Check sheet for the modelled part. Datum: model origin and axes. Units: mm. Round coordinates to 2 decimals unless told otherwise and drop trailing zeros. Write each loop counter-clockwise with the first axis right and the second up, starting at its lowest first coordinate (ties: lowest second). Pieces come first, ordered by that corner, then holes. Notation, with made-up numbers: M -9.75,38.5 L 12.25,38.5 A31 ccw 12.25,65.5 Z; hole C -26.5,56.25 d2. An arc over 180 degrees is marked long. Put each result on its own line as item: value.
```python
from build123d import *

# Parameters (mm, degrees)
F0_R     = 10
F0_R_2   = 8
F1_DEPTH = 100
F4_SIZE  = 1


with BuildPart() as f1:
    # F0 (on Front) → F1 (new body)
    with BuildSketch(Plane.XZ):
        Circle(F0_R)
        Circle(F0_R_2, mode=Mode.SUBTRACT)
    extrude(amount=F1_DEPTH)

    # F2 (on Right) → F3 (revolve)
    with BuildSketch(Plane.YZ):
        Polygon((2, -8), (0, -8), (0, -10), (10, -20), (10, -17.171573), (2, -9.171573), align=None)
    revolve(axis=Axis((0, 7.857602, 0), (0, 1, 0)))

    # F4
    f4_edges = [f1.edges().sort_by_distance(p)[0] for p in [
        (0, 2, 8),
    ]]
    chamfer(f4_edges, length=F4_SIZE)


solid = f1.part
```
1. Cross-section at B-B (x = 0). Enter the section's corners in (y, z), then the cut area to 3 significant figures.
Computed values:
outline: M -100,-10 L 0,-10 L 10,-20 L 10,-17.17 L 2,-9.17 L 2,-9 L 1,-8 L -100,-8 Z; M -100,8 L 1,8 L 2,9 L 2,9.17 L 10,17.17 L 10,20 L 0,10 L -100,10 Z
area: 456 mm2
2. Cross-section at A-A (z = 0). Enter the section's corners in (x, y).
Computed values:
outline: M -20,10 L -10,0 L -10,-100 L -8,-100 L -8,1 L -9,2 L -9.17,2 L -17.17,10 Z; M 8,-100 L 10,-100 L 10,0 L 20,10 L 17.17,10 L 9.17,2 L 9,2 L 8,1 Z
3. Depth check by flat-ended pin: pin 1 Ø1 at (y, z) = (-14, 3.5) entering from +X; pin 2 Ø2 at (x, y) = (5.5, -88.5) entering from -Z; pin 3 Ø2 at (x, z) = (5, -11.5) entering from -Y; pin 4 Ø13 at (x, z) = (0, 0) entering from -Y. Enter the tip coordinate at first touch or a pass-through.
Computed values:
pin 1: stops at x = 9.54
pin 2: stops at z = -8.93
pin 3: stops at y = 1.54
pin 4: passes through
4. Scan lines: probe 1 along Z at (x, y) = (0, 0); probe 2 along X at (y, z) = (-72, -6). Record each from-to range of solid material in increasing order.
Computed values:
probe 1: z = -10 to -8, 8 to 10
probe 2: x = -8 to -5.29, 5.29 to 8
5. Release check for a two-part mould opening along X. For faces 1 (the cylindrical face through (-2.17, -49.3, -9.76)), 2 (the conical face through (-2.87, 2.39, -9.12)), 3 (the flat face through (0, -100, 8.2)) record: +X half, -X half, draft (parallel to the pull), parting line (faces both ways), or undercut.
Computed values:
face 1: parting line
face 2: undercut
face 3: draft
6. Cross-section at C-C (y = -80.5). Enter the section's corners in (x, z), then the cut area to 3 significant figures.
Computed values:
outline: C 0,0 d20; hole C 0,0 d16
area: 113 mm2
